Check sheet for the modelled part. Datum: model origin and axes. Units: mm. A direction names the side the tool comes from. Round coordinates to 2 decimals unless told otherwise and drop trailing zeros. Order: outer loops, then holes, each group sorted by start corner. A loop starts at its lowest first (then second) coordinate and runs counter-clockwise, first axis right, second up. Notation, with made-up numbers: M 27,60 L 45,60 A30 ccw 45,96 Z; hole C 53,58.5 d7. An arc over 180 degrees is marked long. One line per item, written item: value. Start each with the question number.
(1) Depth check by flat-ended pin: pin 1 Ø2 at (x, y) = (-4, 5) entering from -Z; pin 2 Ø1.8 at (x, y) = (4.5, 3) entering from +Z; pin 3 Ø7 at (x, z) = (0, 39.5) entering from +Y; pin 4 Ø1.5 at (x, y) = (41.5, 3) entering from -Z. Enter the tip coordinate at first touch or a pass-through.
(2) Cross-section at B-B, the plane z = 39.5. Enter the section's corners in (x, y).
(3) Thickness scan on L1, parallel to Z at x = 35, y = 4.5; L2, parallel to X at y = 4, z = -3.5; L3, parallel to X at y = 5.75, z = 19.5. Record the ranges inside material, lowest first.
(4) Access from +Z, -Z, +X, -X, +Y, -Y to the whole of each face (thin tool, end or side, straight path). Record for faces 1 (the face through (-4, 4, 53.4)), 2 (the face through (4.28, 4.06, 18.31)), 3 (the face through (-5, 0, -3)), 4 (the face through (5, 4, 50)).
(5) Cross-section at C-C, the plane z = -13.5. Enter the section's corners in (x, y).
(6) Cross-section at D-D, the plane y = 3. Count the separate pieces of the cut face and the enclosed holes in it, and give its area (3 significant figures).
(7) Cross-section at A-A, the plane x = 15. Enter the section's corners in (y, z), and give its area (3 significant figures).
(8) Release check for a two-part mould opening along X. For faces 5 (the face through (-24.384, 4.056, -14.169)), 6 (the face through (0.65, 4.06, 41.55)), 7 (the face through (-2.75, 4, 55)), 8 (the face through (14.96, 4.06, 9.27)) record: released by +X, released by -X, zero draft, split by the parting line, or undercut.
from build123d import *

# Parameters (mm, degrees)
BOSS_EXTRUDE1_DEPTH          = 8
CUT_EXTRUDE1_DEPTH           = 10
ESQUISSE1_W                  = 10
ESQUISSE1_H                  = 25.654784636
BOSS_EXTRU_1_DEPTH           = 8
R_P_TITION_CIRCULAIRE3_COUNT = 3
ESQUISSE3_R                  = 2.15
ENL_V_MAT_EXTRU_1_DEPTH      = 8
BOSS_EXTRU_4_DEPTH           = 8
R_P_TITION_CIRCULAIRE4_COUNT = 3
BOSS_EXTRU_5_DEPTH           = 8
R_P_TITION_CIRCULAIRE5_COUNT = 3
ENL_V_MAT_EXTRU_4_DEPTH      = 10


with BuildPart() as part:
    # Sketch1 → Boss-Extrude1 (new body)
    with BuildSketch(Plane(origin=(0, 0, 0), x_dir=(1, 0, 0), z_dir=(0, 1, 0))):
        Polygon((0, 22.607508486), (-18.985035039, 16.354559035), (-23.655981112, 8.264243118), (-19.578676665, -11.303754243), (-4.670946073, -24.618802154), (4.670946073, -24.618802154), (19.578676665, -11.303754243), (23.655981112, 8.264243118), (18.985035039, 16.354559035), align=None)
        with BuildLine():
            Line((-3.15901992, 5.566021303), (-6.399825806, -0.047219149))
            ThreePointArc((-6.399825806, -0.047219149), (-5.542562584, -3.2), (-3.240805886, -5.518802154))
            Line((-3.240805886, -5.518802154), (3.240805886, -5.518802154))
            ThreePointArc((3.240805886, -5.518802154), (5.542562584, -3.2), (6.399825806, -0.047219149))
            Line((6.399825806, -0.047219149), (3.15901992, 5.566021303))
            ThreePointArc((3.15901992, 5.566021303), (0, 6.4), (-3.15901992, 5.566021303))
        make_face(mode=Mode.SUBTRACT)
    extrude(amount=BOSS_EXTRUDE1_DEPTH)

    # Sketch3 → Cut-Extrude1 (cut)
    with BuildSketch(Plane(origin=(0, 8, 0), x_dir=(1, 0, 0), z_dir=(0, 1, 0))):
        with BuildLine():
            Line((-18.985035039, 16.354559035), (0, 25.029979083))
            Line((0, 25.029979083), (18.985035039, 16.354559035))
            ThreePointArc((18.985035039, 16.354559035), (0, 11.607508486), (-18.985035039, 16.354559035))
        make_face()
        with BuildLine():
            Line((23.655981112, 8.264243118), (24.53433034, -16.532203716))
            Line((24.53433034, -16.532203716), (4.670946073, -24.618802154))
            ThreePointArc((4.670946073, -24.618802154), (10.052397223, -5.803754243), (23.655981112, 8.264243118))
        make_face()
        with BuildLine():
            Line((-23.655981112, 8.264243118), (-26.351688143, -12.502410327))
            Line((-26.351688143, -12.502410327), (-4.670946073, -24.618802154))
            ThreePointArc((-4.670946073, -24.618802154), (-10.052397223, -5.803754243), (-23.655981112, 8.264243118))
        make_face()
    extrude(amount=-CUT_EXTRUDE1_DEPTH, mode=Mode.SUBTRACT)

    # Esquisse1 → Boss.-Extru.1 (add)
    with BuildSketch(Plane.XZ):
        with Locations((0, 33.672607682)):
            Rectangle(ESQUISSE1_W, ESQUISSE1_H)
    boss_extru_1 = extrude(amount=-BOSS_EXTRU_1_DEPTH)

    # R_p_tition circulaire3: Boss.-Extru.1 ×3 about axis
    r_p_tition_circulaire3_axis = Axis((0, 0, 0), (0, 1, 0))
    for i in range(1, R_P_TITION_CIRCULAIRE3_COUNT):
        add(boss_extru_1.rotate(r_p_tition_circulaire3_axis, i * 360 / R_P_TITION_CIRCULAIRE3_COUNT))

    # Esquisse3 → Enl_v. mat.-Extru.1 (cut)
    with BuildSketch(Plane(origin=(0, 8, 0), x_dir=(1, 0, 0), z_dir=(0, 1, 0))):
        with Locations(Location((0, -39.5, 0), (0, 0, 270))):
            Circle(ESQUISSE3_R)
        with Locations(Location((34.208003449, 19.75, 0), (0, 0, 270))):
            Circle(ESQUISSE3_R)
        with Locations(Location((-34.208003449, 19.75, 0), (0, 0, 270))):
            Circle(ESQUISSE3_R)
    extrude(amount=-ENL_V_MAT_EXTRU_1_DEPTH, mode=Mode.SUBTRACT)

    # Esquisse5 → Boss.-Extru.4 (add)
    with BuildSketch(Plane(origin=(0, 8, 0), x_dir=(1, 0, 0), z_dir=(0, 1, 0))):
        with BuildLine():
            Line((-5, -46.5), (5, -46.5))
            Line((5, -46.5), (5, -53.7))
            Line((5, -53.7), (2.75, -53.7))
            Line((2.75, -53.7), (2.75, -56))
            Line((2.75, -56), (4.647580015, -56))
            ThreePointArc((4.647580015, -56), (4.91413701, -56.16235056), (4.89218949, -56.473684211))
            ThreePointArc((4.89218949, -56.473684211), (0, -59), (-4.89218949, -56.473684211))
            ThreePointArc((-4.89218949, -56.473684211), (-4.91413701, -56.16235056), (-4.647580015, -56))
            Line((-4.647580015, -56), (-2.75, -56))
            Line((-2.75, -56), (-2.75, -53.4))
            Line((-2.75, -53.4), (-5, -53.4))
            Line((-5, -53.4), (-5, -46.5))
        make_face()
    boss_extru_4 = extrude(amount=-BOSS_EXTRU_4_DEPTH)

    # R_p_tition circulaire4: Boss.-Extru.4 ×3 about axis
    r_p_tition_circulaire4_axis = Axis((0, 0, 0), (0, 1, 0))
    for i in range(1, R_P_TITION_CIRCULAIRE4_COUNT):
        add(boss_extru_4.rotate(r_p_tition_circulaire4_axis, i * 360 / R_P_TITION_CIRCULAIRE4_COUNT))

    # Esquisse6 → Boss.-Extru.5 (add)
    with BuildSketch(Plane(origin=(0, 8, 0), x_dir=(1, 0, 0), z_dir=(0, 1, 0))):
        with BuildLine():
            Line((4.242203457, -21.192425308), (5, -46.5))
            ThreePointArc((5, -46.5), (15.232576769, -8.794532298), (42.770181276, 18.919872981))
            Line((42.770181276, 18.919872981), (24.63344488, 10.3797127))
            Line((24.63344488, 10.3797127), (9.134543243, -3.221955174))
            Line((9.134543243, -3.221955174), (4.242203457, -21.192425308))
        make_face()
    boss_extru_5 = extrude(amount=-BOSS_EXTRU_5_DEPTH)

    # R_p_tition circulaire5: Boss.-Extru.5 ×3 about axis
    r_p_tition_circulaire5_axis = Axis((0, 0, 0), (0, 1, 0))
    for i in range(1, R_P_TITION_CIRCULAIRE5_COUNT):
        add(boss_extru_5.rotate(r_p_tition_circulaire5_axis, i * 360 / R_P_TITION_CIRCULAIRE5_COUNT))

    # Esquisse12 → Enl_v. mat.-Extru.4 (cut)
    with BuildSketch(Plane(origin=(0, 8, 0), x_dir=(1, 0, 0), z_dir=(0, 1, 0))):
        with BuildLine():
            Line((-7.735382907, 10.239528096), (-19.528767297, 15.41278714))
            ThreePointArc((-19.528767297, 15.41278714), (-24.423894139, 14.101141856), (-23.112248854, 9.206015014))
            Line((-23.112248854, 9.206015014), (-12.735382907, 1.579274058))
            ThreePointArc((-12.735382907, 1.579274058), (-11.113643114, 6.416464843), (-7.735382907, 10.239528096))
        make_face()
        with BuildLine():
            Line((-5, -11.818802154), (-3.583481558, -24.618802154))
            ThreePointArc((-3.583481558, -24.618802154), (0, -28.202283711), (3.583481558, -24.618802154))
            Line((3.583481558, -24.618802154), (5, -11.818802154))
            ThreePointArc((5, -11.818802154), (0, -12.832929687), (-5, -11.818802154))
        make_face()
        with BuildLine():
            Line((12.735382907, 1.579274058), (23.112248854, 9.206015014))
            ThreePointArc((23.112248854, 9.206015014), (24.423894139, 14.101141856), (19.528767297, 15.41278714))
            Line((19.528767297, 15.41278714), (7.735382907, 10.239528096))
            ThreePointArc((7.735382907, 10.239528096), (11.113643114, 6.416464843), (12.735382907, 1.579274058))
        make_face()
    extrude(amount=-ENL_V_MAT_EXTRU_4_DEPTH, mode=Mode.SUBTRACT)


solid = part.part
Values found:
1. pin 1: z = -17.75
1. pin 2: z = 57.8
1. pin 3: y = 8
1. pin 4: z = -30.17
2. outline: M -5.37,0 L -2.15,0 L -2.15,8 L -5.37,8 Z; M 2.15,0 L 5.37,0 L 5.37,8 L 2.15,8 Z
3. L1: -26.08 to -21.75, -17.75 to -13.7
3. L2: -24.06 to -15.35, -12.35 to -4.35, 4.35 to 12.35, 15.35 to 24.06
3. L3: -10.12 to -4.15, 4.15 to 10.12
4. face 1: -X, +Y, -Y
4. face 2: +Y, -Y
4. face 3: +Z, -Z, +X, -X, -Y
4. face 4: +Z, +X, +Y, -Y
5. outline: M -34.74,0 L -24.7,0 L -24.7,8 L -34.74,8 Z; M -15.17,0 L 15.17,0 L 15.17,8 L -15.17,8 Z; M 24.7,0 L 34.74,0 L 34.74,8 L 24.7,8 Z
6. separate pieces: 1
6. enclosed holes: 7
6. area: 2,080 mm^2
7. outline: M 0,-19.08 L 8,-19.08 L 8,-13.43 L 0,-13.43 Z; M 0,-3.24 L 8,-3.24 L 8,9.2 L 0,9.2 Z
7. area: 145 mm^2
8. face 5: undercut
8. face 6: undercut
8. face 7: released by -X
8. face 8: released by +X
